Geometry: final body of the model. Coordinates: model frame, mm. Face numbers are marked on the shaded views. A direction names the side the tool comes from. Round coordinates to 2 decimals unless told otherwise and drop trailing zeros. Loops run counter-clockwise (first coordinate to the right, second up) from the corner with the lowest first, then second, coordinate; pieces in that order, holes last. Notation, with made-up numbers: (82, -38.75) -> (98, -38.75) arc R16 cw to (98, -28.75) -> close; hole circle Ø3 at (62, 68.25). An arc over 180 degrees is marked (long way). Answer in a Markdown table with one row per item.
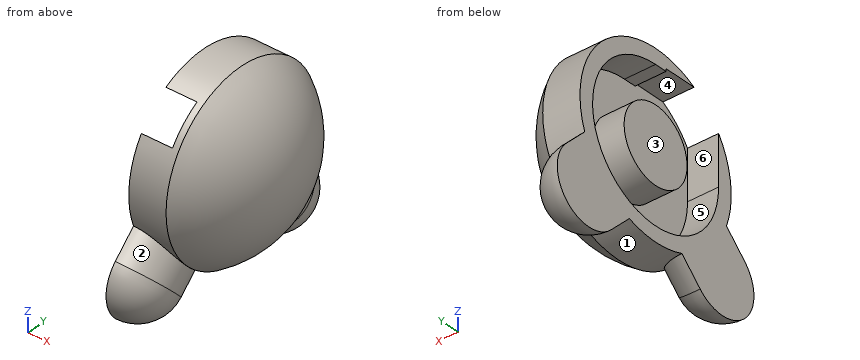
```python
from build123d import *

# Parameters (mm, degrees)
F1_W     = 7.62
F1_H     = 18.288
F4_ANGLE = 180
F5_ANGLE = 180
F0_R     = 7.62
F0_W     = 12.7
F0_H     = 0.508
F6_DEPTH = 6.35


with BuildPart() as f2:
    # F1 (on Front) → F2 (revolve)
    with BuildSketch(Plane.XZ):
        with Locations((3.81, 9.144)):
            Rectangle(F1_W, F1_H)
        with BuildLine():
            ThreePointArc((17.78, 0), (15.0694484018, 10.4603602232), (7.62, 18.288))
            Line((7.62, 18.288), (7.62, 0))
            Line((7.62, 0), (17.78, 0))
        make_face()
    revolve(axis=Axis((3.81, 0, 0), (1, 0, 0)))

    # F3 (on Right) → F4 (revolve)
    with BuildSketch(Plane.YZ):
        Polygon((-16.1644610179, -16.1644610179), (-7.1842048969, -7.1842048969), (-12.5723585695, -1.7960512242), (-21.5526146906, -10.7763073453), align=None)
        with BuildLine():
            Line((-21.5526146906, -21.5526146906), (-16.1644610179, -16.1644610179))
            Line((-16.1644610179, -16.1644610179), (-21.5526146906, -10.7763073453))
            ThreePointArc((-21.5526146906, -10.7763073453), (-23.7844610179, -16.1644610179), (-21.5526146906, -21.5526146906))
        make_face()
    revolve(axis=Axis((0, -8.082230509, -8.082230509), (0, 0.7071067812, 0.7071067812)), revolution_arc=F4_ANGLE)

    # F3 (on Right) → F5 (revolve)
    with BuildSketch(Plane.YZ):
        Polygon((12.5723585695, -1.7960512242), (7.1842048969, -7.1842048969), (16.1644610179, -16.1644610179), (21.5526146906, -10.7763073453), align=None)
        with BuildLine():
            Line((21.5526146906, -10.7763073453), (16.1644610179, -16.1644610179))
            Line((16.1644610179, -16.1644610179), (21.5526146906, -21.5526146906))
            ThreePointArc((21.5526146906, -21.5526146906), (23.7844610179, -16.1644610179), (21.5526146906, -10.7763073453))
        make_face()
    revolve(axis=Axis((0, 8.082230509, -8.082230509), (0, 0.7071067812, -0.7071067812)), revolution_arc=F5_ANGLE)

    # F0 (on Right) → F6 (cut)
    with BuildSketch(Plane.YZ):
        with BuildLine():
            Line((-15.24, 15.24), (-25.4, 15.24))
            Line((-25.4, 15.24), (-25.4, 10.16))
            Line((-25.4, 10.16), (-15.24, 10.16))
            Line((-15.24, 10.16), (-15.24, 0))
            ThreePointArc((-15.24, 0), (10.7763073453, -10.7763073453), (0, 15.24))
            Line((0, 15.24), (-2.54, 15.24))
            Line((-2.54, 15.24), (-15.24, 15.24))
        make_face()
        Circle(F0_R, mode=Mode.SUBTRACT)
        with Locations((-8.89, 15.494)):
            Rectangle(F0_W, F0_H)
    extrude(amount=F6_DEPTH, mode=Mode.SUBTRACT)


solid = f2.part
```
Item 1: Cut plane A-A (x = 3). Output: boundary loops of the cut face in (y, z), then the cut area to 3 significant figures.
Answer:
| item | result |
|---|---|
| outline | (-21.12, -11.21) arc R7 ccw to (-11.21, -21.12) -> (-6.99, -16.9) arc R18.29 ccw to (6.99, -16.9) -> (11.21, -21.12) arc R7 ccw to (21.12, -11.21) -> (16.9, -6.99) arc R18.29 ccw to (-9.3, 15.75) -> (-2.54, 15.75) -> (-2.54, 15.24) -> (0, 15.24) arc R15.24 cw (long way) to (-15.24, 0) -> (-15.24, 10.11) arc R18.29 ccw to (-16.9, -6.99) -> close; circle Ø15.24 at (0, 0) |
| area | 756 mm² |
Item 2: Cut plane C-C (y = -2). Output: boundary loops of the cut face in (x, z), then the cut area to 3 significant figures.
Answer:
| item | result |
|---|---|
| outline | (0, -18.18) -> (7.62, -18.18) arc R21.45 ccw to (7.62, 18.18) -> (0, 18.18) -> (0, 15.24) -> (6.35, 15.24) -> (6.35, 7.35) -> (0, 7.35) -> (0, -7.35) -> (6.35, -7.35) -> (6.35, -15.11) -> (0, -15.11) -> close |
| area | 436 mm² |
Item 3: Pin query (flat end, axial travel): pin 1 Ø3 at (x, z) = (2.5, 5) entering from +Y; pin 2 Ø5 at (x, y) = (3.5, -4.5) entering from -Z; pin 3 Ø4 at (y, z) = (14, -13) entering from +X. Return the tip coordinate at first contact, or that it passes through.
Answer:
| item | result |
|---|---|
| pin 1 | stops at y = 17.95 |
| pin 2 | stops at z = -18.18 |
| pin 3 | stops at x = 9.33 |
Item 4: Draft query along Z for the marked faces 1, 2 and 3. Return one class per face: pulls with the +Z half, pulls with the -Z half, needs draft (parallel to the pull), parting line crosses it, or undercut.
Answer:
| item | result |
|---|---|
| face 1 | pulls with the -Z half |
| face 2 | undercut |
| face 3 | needs draft |
Item 5: Reachability of the marked faces 4, 5 and 6 from +Z, -Z, +X, -X, +Y, -Y: full face, straight path, thin tool, end or side. Return the list, or none.
Answer:
| item | result |
|---|---|
| face 4 | -X, -Y |
| face 5 | -X |
| face 6 | +Z, -X |
Item 6: Cut plane B-B (z = 8.5). Output: boundary loops of the cut face in (x, y), then the cut area to 3 significant figures.
Answer:
| item | result |
|---|---|
| outline | (0, -16.19) -> (7.62, -16.19) arc R19.79 ccw to (7.62, 16.19) -> (0, 16.19) -> (0, 12.65) -> (6.35, 12.65) -> (6.35, -15.24) -> (0, -15.24) -> close |
| area | 261 mm² |
Item 7: Line query: probe 1 along Z at (x, y) = (1.5, 0); probe 2 along Y at (x, z) = (3, -5); probe 3 along Y at (x, z) = (3, -4.5). Output: solid intervals per line, ascending. Write a range as [from, to].
Answer:
| item | result |
|---|---|
| probe 1 | z = [-18.29, -15.24], [-7.62, 7.62], [15.24, 18.29] |
| probe 2 | y = [-17.59, -14.4], [-5.75, 5.75], [14.4, 17.59] |
| probe 3 | y = [-17.73, -14.56], [-6.15, 6.15], [14.56, 17.73] |
